CAD build for the part. Positions are in the model's coordinates, mm. Face numbers are marked on the shaded views. Coordinates: 2 decimals unless noted, no trailing zeros. Write each loop counter-clockwise with the first axis right and the second up, starting at its lowest first coordinate (ties: lowest second). Pieces come first, ordered by that corner, then holes. Notation, with made-up numbers: (65, 69.5) - (106, 69.5) arc R23 cw to (106, 83.5) - close; hole circle Ø1 at (23, 70). An arc over 180 degrees is marked (long way). One line per question, with ' | ' between items. Start each with the question number.
1. Two-plate mould, pull along Y, no slides. Class the marked faces 1, 2 and 3: +Y half, -Y half, draft (parallel to the pull), parting line (faces both ways), or undercut.
2. Probe line 1 (Y direction, x = 0, z = 3.25); line 2 (Y direction, x = -20, z = 4.5); line 3 (X direction, y = 11.5, z = 6.25). List the from-to ranges inside material, lowest first.
3. Band-saw the part on B-B, the plane y = 0. Write the cut outline in (x, z), then the cut area to 3 significant figures.
4. Band-saw the part on C-C, the plane x = 21. Give the number of separate pieces and of enclosed holes in the cut face, then the cut area to 3 significant figures.
5. Flat gauge pins, fed straight in: P1, Ø1.5, axis at x = -20, z = 2, coming from the -Y side; P2, Ø1, axis at x = 3, z = 5, coming from the +Y side. Where does each tip first touch, or does it go through?
6. Band-saw the part on A-A, the plane x = 0. Write the cut outline in (y, z), then the cut area to 3 significant figures.
from build123d import *

# Parameters (mm, degrees)
SKETCH1_R           = 30.9372
SKETCH1_R_2         = 2.032
SKETCH1_R_3         = 16.7132
BOSS_EXTRUDE1_DEPTH = 6.35
CHAMFER1_SIZE       = 0.79375


with BuildPart() as part:
    # Sketch1 → Boss-Extrude1 (new body)
    with BuildSketch(Plane.XY):
        Circle(SKETCH1_R)
        with Locations((0, 23.8252)):
            Circle(SKETCH1_R_2, mode=Mode.SUBTRACT)
        Circle(SKETCH1_R_3, mode=Mode.SUBTRACT)
        with Locations((20.63322845, 11.9126)):
            Circle(SKETCH1_R_2, mode=Mode.SUBTRACT)
        with Locations((20.63322845, -11.9126)):
            Circle(SKETCH1_R_2, mode=Mode.SUBTRACT)
        with Locations((0, -23.8252)):
            Circle(SKETCH1_R_2, mode=Mode.SUBTRACT)
        with Locations((-20.63322845, -11.9126)):
            Circle(SKETCH1_R_2, mode=Mode.SUBTRACT)
        with Locations((-20.63322845, 11.9126)):
            Circle(SKETCH1_R_2, mode=Mode.SUBTRACT)
    extrude(amount=BOSS_EXTRUDE1_DEPTH)

    # Chamfer1
    chamfer1_edges = [part.edges().sort_by_distance(p)[0] for p in [
        (-30.9372, 0, 0),
        (-30.9372, 0, 6.35),
        (-16.7132, 0, 0),
        (-16.7132, 0, 6.35),
    ]]
    chamfer(chamfer1_edges, length=CHAMFER1_SIZE)


solid = part.part
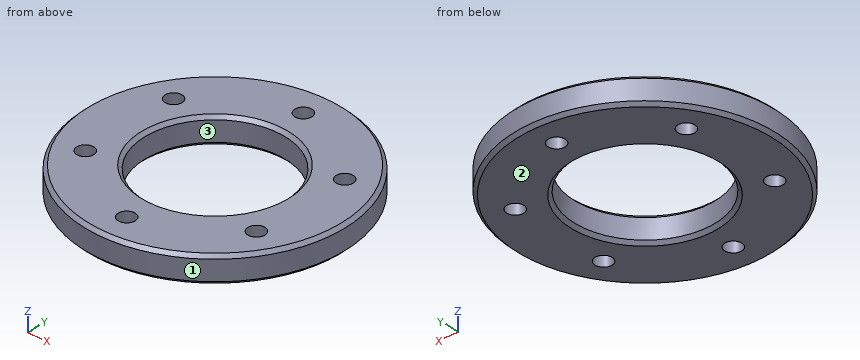
Filled in:
1) face 1: parting line | face 2: draft | face 3: undercut
2) line 1: y = -30.94 to -25.86, -21.79 to -16.71, 16.71 to 21.79, 25.86 to 30.94 | line 2: y = -23.6 to -13.84, -9.98 to 9.98, 13.84 to 23.6 | line 3: x = -27.97 to -22.62, -18.64 to -13.07, 13.07 to 18.64, 22.62 to 27.97
3) outline: (-30.94, 0.79) - (-30.14, 0) - (-17.51, 0) - (-16.71, 0.79) - (-16.71, 5.56) - (-17.51, 6.35) - (-30.14, 6.35) - (-30.94, 5.56) - close; (16.71, 0.79) - (17.51, 0) - (30.14, 0) - (30.94, 0.79) - (30.94, 5.56) - (30.14, 6.35) - (17.51, 6.35) - (16.71, 5.56) - close | area: 178 mm²
4) separate pieces: 3 | enclosed holes: 0 | area: 236 mm²
5) P1: stops at y = -24.22 | P2: stops at y = 30.84
6) outline: (-30.94, 0.79) - (-30.14, 0) - (-25.86, 0) - (-25.86, 6.35) - (-30.14, 6.35) - (-30.94, 5.56) - close; (-21.79, 0) - (-17.51, 0) - (-16.71, 0.79) - (-16.71, 5.56) - (-17.51, 6.35) - (-21.79, 6.35) - close; (16.71, 0.79) - (17.51, 0) - (21.79, 0) - (21.79, 6.35) - (17.51, 6.35) - (16.71, 5.56) - close; (25.86, 0) - (30.14, 0) - (30.94, 0.79) - (30.94, 5.56) - (30.14, 6.35) - (25.86, 6.35) - close | area: 127 mm²
